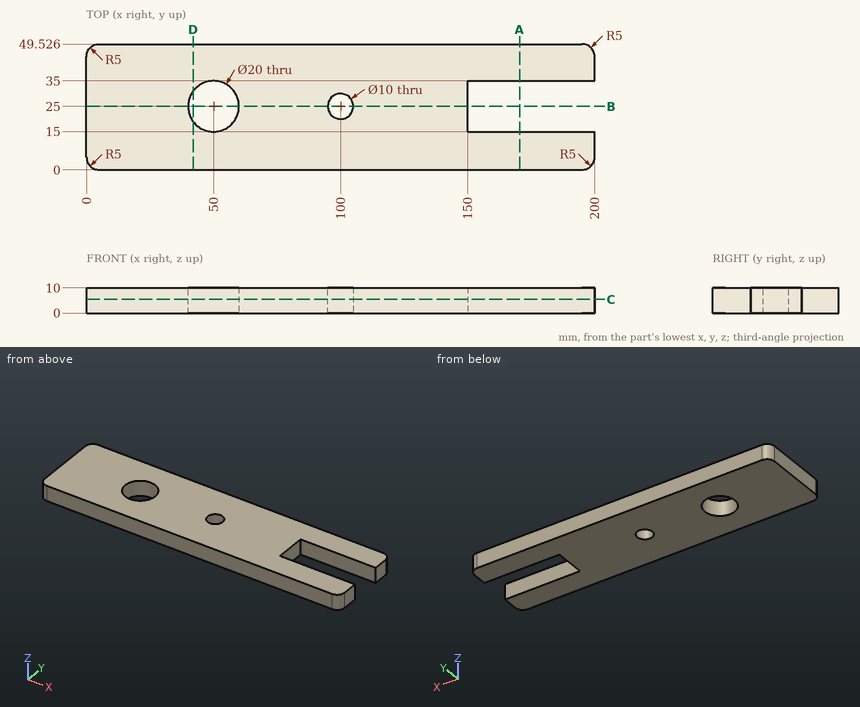
The drawing under review shows one solid part. Ordinate dimensions are in mm from its lowest x, y, z. Round coordinates to 2 decimals unless told otherwise and drop trailing zeros. Loops run counter-clockwise (first coordinate to the right, second up) from the corner with the lowest first, then second, coordinate; pieces in that order, holes last. Notation, with made-up numbers: (65, 22) -> (96, 22) arc R21 ccw to (96, 36) -> close; hole circle Ø4 at (29, 27). An arc over 180 degrees is marked (long way). Answer in a Markdown table with one row per item.
1) Consider section D-D, the plane x = 42. Write out the cut boundary in (y, z), plus the area to 3 significant figures.
Taken from the geometry:
| item | result |
|---|---|
| outline | (0, 0) -> (19, 0) -> (19, 10) -> (0, 10) -> close; (31, 0) -> (49.53, 0) -> (49.53, 10) -> (31, 10) -> close |
| area | 375 mm² |
2) Consider section B-B, the plane y = 25. Write out the cut boundary in (x, z).
Taken from the geometry:
| item | result |
|---|---|
| outline | (0, 0) -> (40, 0) -> (40, 10) -> (0, 10) -> close; (60, 0) -> (95, 0) -> (95, 10) -> (60, 10) -> close; (105, 0) -> (150, 0) -> (150, 10) -> (105, 10) -> close |
3) Wall thickness on line 1 along X through (y, z) = (24.5, 1.25) (1 decimal); line 2 along Y through (x, z) = (163, 6.25); line 3 along Y through (x, z) = (100, 8.25): over which ranges is each line inside the solid? List them lowest first.
Taken from the geometry:
| item | result |
|---|---|
| line 1 | x = 0 to 40, 60 to 95, 105 to 150 |
| line 2 | y = 0 to 15, 35 to 49.53 |
| line 3 | y = 0 to 20, 30 to 49.53 |
4) Consider section C-C, the plane z = 5.5. Write out the cut boundary in (x, y).
Taken from the geometry:
| item | result |
|---|---|
| outline | (0, 5) arc R5 ccw to (5, 0) -> (195, 0) arc R5 ccw to (200, 5) -> (200, 15) -> (150, 15) -> (150, 35) -> (200, 35) -> (200, 44.53) arc R5 ccw to (195, 49.53) -> (5, 49.53) arc R5 ccw to (0, 44.53) -> close; hole circle Ø20 at (50, 25); hole circle Ø10 at (100, 25) |
5) Consider section A-A, the plane x = 170.5. Write out the cut boundary in (y, z).
Taken from the geometry:
| item | result |
|---|---|
| outline | (0, 0) -> (15, 0) -> (15, 10) -> (0, 10) -> close; (35, 0) -> (49.53, 0) -> (49.53, 10) -> (35, 10) -> close |
